Source: CAD feature listing. Evaluate the final solid. Frame: model axes, mm. A direction names the side the tool comes from. Give positions to 0.01 mm unless a question says otherwise; leave off trailing zeros. Write each loop counter-clockwise with the first axis right and the second up, starting at its lowest first coordinate (ties: lowest second). Pieces come first, ordered by that corner, then holes. Notation, with made-up numbers: (58.25, -11.75) - (99.25, -11.75) arc R22 cw to (99.25, 24.25) - close; hole circle Ø4 at (87.5, 52.5). An arc over 180 degrees is marked (long way). Answer as a JSON object with one key per item and string values. Group by question number.
from build123d import *

# Parameters (mm, degrees)
F0_W     = 60
F0_H     = 550
F1_DEPTH = 2
F2_W     = 38
F2_H     = 550
F2_W_2   = 2
F3_DEPTH = 2
F4_W     = 38
F4_H     = 550
F4_W_2   = 2
F5_DEPTH = 2
F6_R     = 1.5
F7_R     = 1.5
F8_R     = 4
F9_DEPTH = 64.001


with BuildPart() as f1:
    # F0 (on Front) → F1 (new body)
    with BuildSketch(Plane.XZ):
        with Locations((-30, 275)):
            Rectangle(F0_W, F0_H)
    extrude(amount=-F1_DEPTH)

    # F2 (on face) → F3 (join)
    with BuildSketch(Plane.YZ):
        with Locations((-19, 275)):
            Rectangle(F2_W, F2_H)
        with Locations((1, 275)):
            Rectangle(F2_W_2, F2_H)
    extrude(amount=F3_DEPTH)

    # F4 (on face) → F5 (join)
    with BuildSketch(Plane(origin=(-60, 0, 0), x_dir=(0, -1, 0), z_dir=(-1, 0, 0))):
        with Locations((19, 275)):
            Rectangle(F4_W, F4_H)
        with Locations((-1, 275)):
            Rectangle(F4_W_2, F4_H)
    extrude(amount=F5_DEPTH)

    # F6
    f6_edges = [f1.edges().sort_by_distance(p)[0] for p in [
        (-61, -38, 0),
        (1, -38, 0),
    ]]
    fillet(f6_edges, radius=F6_R)

    # F7
    f7_edges = [f1.edges().sort_by_distance(p)[0] for p in [
        (-61, -38, 550),
        (1, -38, 550),
    ]]
    fillet(f7_edges, radius=F7_R)

    # F8 (on face) → F9 (cut, through all)
    with BuildSketch(Plane(origin=(-62, 0, 0), x_dir=(0, -1, 0), z_dir=(-1, 0, 0))):
        with Locations((26, 312)):
            Circle(F8_R)
        with Locations((26, 34)):
            Circle(F8_R)
    extrude(amount=-F9_DEPTH, mode=Mode.SUBTRACT)


solid = f1.part
Q1. Draft query along X for faces 3 (the flat face through (-30, 1, 550)), 4 (the flat face through (-60, -19, 279)), 5 (the flat face through (-62, -18, 279)), 6 (the flat face through (-30, 0, 279)). Return one class per face: released by +X, released by -X, zero draft, split by the parting line, or undercut.
Q2. Reachability of faces 1 (the flat face through (-30, 2, 271)), 2 (the flat face through (0, -19, 279)) from +Z, -Z, +X, -X, +Y, -Y: full face, straight path, thin tool, end or side. Return the list, or none.
Q3. Section C-C on x = -9. Return the cut outline in (y, z), then the cut area to 3 significant figures.
Q4. Ray query, probe 1 along Z at (x, y) = (1.55, -26); probe 2 along X at (y, z) = (-27.5, 288.5); probe 3 along Y at (x, z) = (-61.55, 312). Return the intervals inside material, ascending. Write a range as [from, to].
Q5. First-contact query: pin 1 Ø6 at (x, y) = (-5.5, -23) entering from +Z; pin 2 Ø18 at (x, z) = (-32.5, 300) entering from -Y. Flat tips, straight axial feed; report the tip coordinate or a pass-through.
Q6. Section A-A on y = -16. Return the cut outline in (x, z), then the cut area to 3 significant figures.
Q7. Section B-B on z = 396. Return the cut outline in (x, y), then the cut area to 3 significant figures.
Taken from the geometry:
{
 "1": {"face 3": "zero draft", "face 4": "undercut", "face 5": "released by -X", "face 6": "undercut"},
 "2": {"face 1": "+Z, -Z, +X, -X, +Y", "face 2": "+Z, -Z, -Y"},
 "3": {"outline": "(0, 0) - (2, 0) - (2, 550) - (0, 550) - close", "area": "1,100 mm²"},
 "4": {"probe 1": "z = [0, 30], [38, 308], [316, 550]", "probe 2": "x = [-62, -60], [0, 2]", "probe 3": "y = [-38, -30], [-22, 2]"},
 "5": {"pin 1": "passes through", "pin 2": "stops at y = 0"},
 "6": {"outline": "(-62, 0) - (-60, 0) - (-60, 550) - (-62, 550) - close; (0, 0) - (2, 0) - (2, 550) - (0, 550) - close", "area": "2,200 mm²"},
 "7": {"outline": "(-62, -38) - (-60, -38) - (-60, 0) - (0, 0) - (0, -38) - (2, -38) - (2, 2) - (-62, 2) - close", "area": "280 mm²"}
}
